```python
from build123d import *

# Parameters (mm, degrees)
BOSS_EXTRUDE1_DEPTH = 10
EXTRUDE_THIN1_DEPTH = 20
CHAMFER1_SIZE       = 10
SKETCH4_W           = 5
SKETCH4_H           = 8
CUT_EXTRUDE1_DEPTH  = 99


with BuildPart() as part:
    # Sketch1 → Boss-Extrude1 (new body)
    with BuildSketch(Plane(origin=(0, 0, 0), x_dir=(1, 0, 0), z_dir=(0, 1, 0))):
        Polygon((0, 39.088250925), (0, 0), (63.815145827, 0), (63.815145827, 46), (26, 46), (26, 86), (0, 86), align=None)
    extrude(amount=BOSS_EXTRUDE1_DEPTH)

    # Sketch2 → Extrude-Thin1 (add)
    with BuildSketch(Plane(origin=(0, 10, 0), x_dir=(1, 0, 0), z_dir=(0, 1, 0))):
        Polygon((0, 86), (0, 0), (63.815145827, 0), (63.815145827, 3), (3, 3), (3, 86), align=None)
        Polygon((63.815145827, 46), (26, 46), (26, 86), (23, 86), (23, 43), (63.815145827, 43), align=None)
    extrude(amount=EXTRUDE_THIN1_DEPTH)

    # Chamfer1
    chamfer1_edges = [part.edges().sort_by_distance(p)[0] for p in [
        (63.815145827, 30, -1.5),
        (1.5, 30, -86),
    ]]
    chamfer(chamfer1_edges, length=CHAMFER1_SIZE)

    # Sketch4 → Cut-Extrude1 (cut)
    with BuildSketch(Plane.XY):
        with Locations((12.4, 5)):
            Rectangle(SKETCH4_W, SKETCH4_H)
        with Locations((4.5, 5)):
            Rectangle(SKETCH4_W, SKETCH4_H)
        with Locations((20.3, 5)):
            Rectangle(SKETCH4_W, SKETCH4_H)
        with Locations((28.2, 5)):
            Rectangle(SKETCH4_W, SKETCH4_H)
        with Locations((36.1, 5)):
            Rectangle(SKETCH4_W, SKETCH4_H)
        with Locations((44, 5)):
            Rectangle(SKETCH4_W, SKETCH4_H)
        with Locations((51.9, 5)):
            Rectangle(SKETCH4_W, SKETCH4_H)
        with Locations((59.8, 5)):
            Rectangle(SKETCH4_W, SKETCH4_H)
    extrude(amount=-CUT_EXTRUDE1_DEPTH, mode=Mode.SUBTRACT)


solid = part.part
```
Verification items for the finished model (mm, model axes). A direction names the side the tool comes from. Coordinates: 2 decimals unless noted, no trailing zeros. Order: outer loops, then holes, each group sorted by start corner. A loop starts at its lowest first (then second) coordinate and runs counter-clockwise, first axis right, second up. Notation, with made-up numbers: (28.5, 86.5) -> (48.5, 86.5) arc R15 ccw to (48.5, 90.5) -> close; hole circle Ø8 at (-40, 13.5). An arc over 180 degrees is marked (long way). Put each result on its own line as item: value. Start each with the question number.
1) Tool access check on faces 4 (the flat face through (60, 1, -23)), 5 (the flat face through (58.745, 25.07, -1.479)), 6 (the flat face through (3, 20, -44)), 7 (the flat face through (24, 0, -34)). Record the directions out of +Z, -Z, +X, -X, +Y, -Y that give a thin tool (end or side, any length) a straight path to the whole face; none if there is none.
2) Material ranges on L1, parallel to X at y = 3.75, z = -47.5; L2, parallel to Z at x = 37.5, y = 25.5; L3, parallel to Y at x = 30, z = -25, recorded low to high.
3) Cross-section at D-D (x = 32). Enter the section's corners in (y, z), plus the area to 3 significant figures.
4) Cross-section at C-C (y = 22). Enter the section's corners in (x, z).
5) Cross-section at B-B (z = -73.5). Enter the section's corners in (x, y), plus the area to 3 significant figures.
6) Go/stop test with flat-tipped pins: pin 1 (1.5 mm diameter, centred on x = 11.5, z = -41.5, fed in from -Y); pin 2 (6.5 mm diameter, centred on y = 20.5, z = -66.5, fed in from +X); pin 3 (5.5 mm diameter, centred on x = 13.5, z = -63, fed in from +Y); pin 4 (1.5 mm diameter, centred on x = 29.5, z = -48.5, fed in from -Y). Record where each tip stops, or that it passes through.
7) Cross-section at A-A (x = 45). Enter the section's corners in (y, z), plus the area to 3 significant figures.
8) Release check for a two-part mould opening along Z. For faces 1 (the flat face through (15, 9.4, -86)), 2 (the flat face through (4, 9, -42)), 3 (the flat face through (43, 20, -43)) record: pulls with the +Z half, pulls with the -Z half, needs draft (parallel to the pull), parting line crosses it, or undercut.
Geometry check:
1. face 4: +Z, -Z
1. face 5: +Z, +X, +Y
1. face 6: -Z, +Y
1. face 7: +Z, -Z, +X, -X, -Y
2. L1: x = 0 to 2, 7 to 9.9, 14.9 to 17.8, 22.8 to 25.7
2. L2: z = -46 to -43, -3 to 0
2. L3: y = 0 to 1, 9 to 10
3. outline: (0, -46) -> (30, -46) -> (30, -43) -> (10, -43) -> (10, -3) -> (30, -3) -> (30, 0) -> (0, 0) -> close
3. area: 580 mm^2
4. outline: (0, -84) -> (3, -84) -> (3, -3) -> (61.82, -3) -> (61.82, 0) -> (0, 0) -> close; (23, -86) -> (26, -86) -> (26, -46) -> (63.82, -46) -> (63.82, -43) -> (23, -43) -> close
5. outline: (0, 0) -> (26, 0) -> (26, 1) -> (25.7, 1) -> (25.7, 9) -> (26, 9) -> (26, 30) -> (23, 30) -> (23, 10) -> (3, 10) -> (3, 30) -> (0, 30) -> close; hole (2, 1) -> (7, 1) -> (7, 9) -> (2, 9) -> close; hole (9.9, 1) -> (14.9, 1) -> (14.9, 9) -> (9.9, 9) -> close; hole (17.8, 1) -> (22.8, 1) -> (22.8, 9) -> (17.8, 9) -> close
5. area: 258 mm^2
6. pin 1: stops at y = 0
6. pin 2: stops at x = 26
6. pin 3: stops at y = 10
6. pin 4: passes through
7. outline: (0, -46) -> (1, -46) -> (1, 0) -> (0, 0) -> close; (9, -46) -> (30, -46) -> (30, -43) -> (10, -43) -> (10, -3) -> (30, -3) -> (30, 0) -> (9, 0) -> close
7. area: 212 mm^2
8. face 1: pulls with the -Z half
8. face 2: needs draft
8. face 3: undercut
